Part model, mm, in its own coordinate system. A direction names the side the tool comes from. Round coordinates to 2 decimals unless told otherwise and drop trailing zeros. Loops run counter-clockwise (first coordinate to the right, second up) from the corner with the lowest first, then second, coordinate; pieces in that order, holes last. Notation, with made-up numbers: M 77,63 L 98,63 A20 cw 98,98 Z; hole C 73.5,48 d5. An arc over 180 degrees is marked long. Put each result on its own line as item: value. Start each with the question number.
1) Which spindle directions (+Z, -Z, +X, -X, +Y, -Y) get a long thin tool onto all of the face, cutting with end or side? Do faces 1 (the flat face through (4, 10.1, 0)), 2 (the cylindrical face through (2.205, 11.538, 12.325)). Say none if no direction does.
2) Drop flat-ended pins along their axis: pin 1 Ø2 at (y, z) = (3, 9.5) entering from +X; pin 2 Ø12 at (x, z) = (6.5, 3) entering from +Y; pin 3 Ø2 at (y, z) = (15, 18) entering from -X. Give the stop position or say it passes through.
3) Probe line 1 along Z through (x, y) = (9, 22); line 2 along X through (y, z) = (10.5, 1.75); line 3 along X through (y, z) = (6.75, 11). List the from-to ranges inside material, lowest first.
4) Slice it at A-A on z = 5. Give the cut face in (x, y), then the cut area to 3 significant figures.
```python
from build123d import *

# Parameters (mm, degrees)
F1_ANGLE    = 90
F2_R        = 1.5
F3_T2_ANGLE = 120.4977458854
F4_R        = 2


# Not quite as in the source:
# - a fillet or chamfer that OpenCascade refuses, or shapes differently, is made with other operations: its cross-section is extruded or revolved along the edge and cut away or added


with BuildPart() as f1:
    # F0 (on Front) → F1 (revolve)
    with BuildSketch(Plane.XZ):
        Polygon((-2.5, 0), (0, 0), (0, 28), (-15, 28), (-15, 25), (-12.5, 25), (-2.5, 25), align=None)
    revolve(axis=Axis((14, 0, -3.1492561102), (0, 0, -1)), revolution_arc=F1_ANGLE)

    # F2
    f2_edges = [f1.edges().sort_by_distance(p)[0] for p in [
        (-6.506097, 20.506097, 25),
    ]]
    fillet(f2_edges, radius=F2_R)

    # F3: chamfer of 3 on 1 edges, made by hand

    # F3_s1 → F3_t2 (revolve, cut)
    with BuildSketch(Plane(origin=(0.9684561095, -3.5525312522, 0), x_dir=(0, 0, 1), z_dir=(0.2630122362, -0.9647924977, 0))):
        Polygon((25, 15.4929050323), (28, 12.4929050323), (28, 15.4929050323), align=None)
    revolve(axis=Axis((14, 0, 28), (0, 0, -1)), revolution_arc=F3_T2_ANGLE, mode=Mode.SUBTRACT)

    # F4
    f4_edges = [f1.edges().sort_by_distance(p)[0] for p in [
        (4.100505, 9.899495, 28),
    ]]
    fillet(f4_edges, radius=F4_R)


solid = f1.part
```
Recorded:
1. face 1: -Z, +X, -X, +Y, -Y
1. face 2: -Z, -X, +Y
2. pin 1: stops at x = 0.58
2. pin 2: stops at y = 16.43
2. pin 3: stops at x = 5.27
3. line 1: z = 25 to 28
3. line 2: x = 1.27 to 4.74
3. line 3: x = -1.06 to 1.73
4. outline: M -2.5,0 L 0,0 A14 cw 14,14 L 14,16.5 A16.5 ccw Z
4. area: 59.9 mm2
